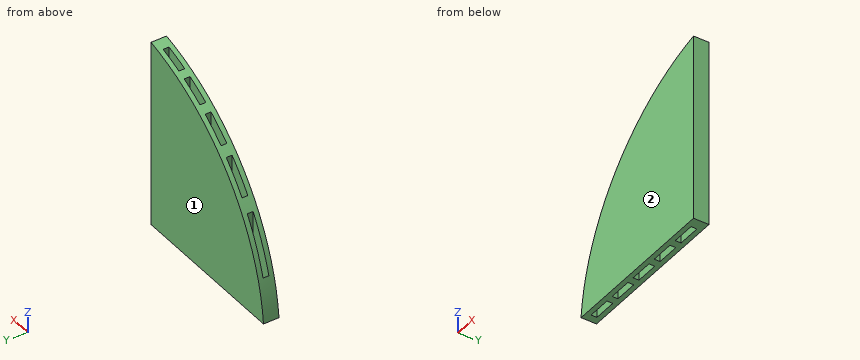
```python
from build123d import *

# Parameters (mm, degrees)
F1_DEPTH = 2
F2_W     = 3
F2_H     = 0.75
F3_DEPTH = 25


with BuildPart() as f1:
    # F0 (on Front) → F1 (new body)
    with BuildSketch(Plane.XZ):
        with BuildLine():
            Line((-6, 2.5), (-6, 26.837474))
            ThreePointArc((-6, 26.837474), (-20.657603, 18.152506), (-27.386128, 2.5))
            Line((-27.386128, 2.5), (-6, 2.5))
        make_face()
    extrude(amount=F1_DEPTH)

    # F2 (on face) → F3 (cut)
    with BuildSketch(Plane(origin=(0, 0, 2.5), x_dir=(1, 0, 0), z_dir=(0, 0, -1))):
        with Locations((-24.886128, 1)):
            Rectangle(F2_W, F2_H)
        with Locations((-20.886128, 1)):
            Rectangle(F2_W, F2_H)
        with Locations((-16.886128, 1)):
            Rectangle(F2_W, F2_H)
        with Locations((-12.886128, 1)):
            Rectangle(F2_W, F2_H)
        with Locations((-8.886128, 1)):
            Rectangle(F2_W, F2_H)
    extrude(amount=-F3_DEPTH, mode=Mode.SUBTRACT)


solid = f1.part
```
Source: CAD feature listing. Evaluate the final solid. Frame: model axes, mm. Face numbers are marked on the shaded views. Coordinates: 2 decimals unless noted, no trailing zeros. Loops run counter-clockwise (first coordinate to the right, second up) from the corner with the lowest first, then second, coordinate; pieces in that order, holes last. Notation, with made-up numbers: (-32, -4.5) -> (11, -4.5) arc R24 cw to (11, 20.5) -> close; hole circle Ø9 at (-21, 3). An arc over 180 degrees is marked (long way). One line per item, written item: value. Start each with the question number.
Q1. Section query D-D, the plane z = 23.75. Return the cut outline in (x, y) (3 decimals), and give its area (3 significant figures).
Q2. Mould query, pull axis Y, two halves, no side actions, for the marked faces 1 and 2. Classes: pulls with the +Y half, pulls with the -Y half, needs draft (parallel to the pull), parting line crosses it, or undercut.
Q3. Line query: line 1 along X through (y, z) = (-1, 8.25); line 2 along Y through (x, z) = (-10.25, 18) (3 decimals); line 3 along X through (y, z) = (-0.9, 15.75). Output: solid intervals per line, ascending.
Q4. Section query C-C, the plane z = 7. Return the cut outline in (x, y) (3 decimals).
Q5. Section query B-B, the plane y = -1.1. Return the cut outline in (x, z), and give its area (3 significant figures).
Q6. Section query A-A, the plane x = -16.5. Return the cut outline in (y, z) (3 decimals), and give its area (3 significant figures).
Q7. Contact query for flat-ended pins moving along their axis: P1, Ø0.6, axis at y = -1, z = 13.5, coming from the -X side; P2, Ø1, axis at y = -1.5, z = 22.5, coming from the -X side. Output: stop coordinate, or through.
Results:
1. outline: (-13.863, -2) -> (-6, -2) -> (-6, 0) -> (-13.863, 0) -> (-13.863, -0.625) -> (-11.386, -0.625) -> (-11.386, -1.375) -> (-13.863, -1.375) -> close; hole (-10.386, -1.375) -> (-7.386, -1.375) -> (-7.386, -0.625) -> (-10.386, -0.625) -> close
1. area: 11.6 mm^2
2. face 1: pulls with the +Y half
2. face 2: pulls with the -Y half
3. line 1: -23.39 to -22.39, -19.39 to -18.39, -15.39 to -14.39, -11.39 to -10.39, -7.39 to -6
3. line 2: -2 to -1.375, -0.625 to 0
3. line 3: -22.54 to -22.39, -19.39 to -18.39, -15.39 to -14.39, -11.39 to -10.39, -7.39 to -6
4. outline: (-26.594, -2) -> (-6, -2) -> (-6, 0) -> (-26.594, 0) -> close; hole (-26.386, -1.375) -> (-23.386, -1.375) -> (-23.386, -0.625) -> (-26.386, -0.625) -> close; hole (-22.386, -1.375) -> (-19.386, -1.375) -> (-19.386, -0.625) -> (-22.386, -0.625) -> close; hole (-18.386, -1.375) -> (-15.386, -1.375) -> (-15.386, -0.625) -> (-18.386, -0.625) -> close; hole (-14.386, -1.375) -> (-11.386, -1.375) -> (-11.386, -0.625) -> (-14.386, -0.625) -> close; hole (-10.386, -1.375) -> (-7.386, -1.375) -> (-7.386, -0.625) -> (-10.386, -0.625) -> close
5. outline: (-27.39, 2.5) -> (-26.39, 2.5) -> (-26.39, 7.75) arc R27.5 ccw to start; (-23.39, 2.5) -> (-22.39, 2.5) -> (-22.39, 15.97) arc R27.5 ccw to (-23.39, 14.47) -> close; (-19.39, 2.5) -> (-18.39, 2.5) -> (-18.39, 20.45) arc R27.5 ccw to (-19.39, 19.5) -> close; (-15.39, 2.5) -> (-14.39, 2.5) -> (-14.39, 23.44) arc R27.5 ccw to (-15.39, 22.79) -> close; (-11.39, 2.5) -> (-10.39, 2.5) -> (-10.39, 25.46) arc R27.5 ccw to (-11.39, 25.03) -> close; (-7.39, 2.5) -> (-6, 2.5) -> (-6, 26.84) arc R27.5 ccw to (-7.39, 26.49) -> close
5. area: 110 mm^2
6. outline: (-2, 2.5) -> (-1.375, 2.5) -> (-1.375, 22) -> (-2, 22) -> close; (-0.625, 2.5) -> (0, 2.5) -> (0, 22) -> (-0.625, 22) -> close
6. area: 24.4 mm^2
7. P1: x = -23.39
7. P2: x = -16.5
